CAD build for the part. Positions are in the model's coordinates, mm. A direction names the side the tool comes from. Coordinates: 2 decimals unless noted, no trailing zeros. Write each loop counter-clockwise with the first axis right and the second up, starting at its lowest first coordinate (ties: lowest second). Pieces come first, ordered by that corner, then holes.
```python
from build123d import *

# Parameters (mm, degrees)
F0_W     = 30
F0_H     = 4.3
F1_DEPTH = 4.3
F2_W     = 4
F2_H     = 2.3
F6_DEPTH = 4.301
F3_SIZE  = 0.25
F4_R     = 1.5
F5_DEPTH = 23


with BuildPart() as f1:
    # F0 (on Top) → F1 (new body)
    with BuildSketch(Plane.XY):
        with Locations((-1.762214, 2.15)):
            Rectangle(F0_W, F0_H)
    extrude(amount=F1_DEPTH)

    # F2 (on face) → F6 (cut, through all)
    with BuildSketch(Plane.XY.offset(4.3)):
        with Locations((9.737786, 2.15)):
            Rectangle(F2_W, F2_H)
    extrude(amount=-F6_DEPTH, mode=Mode.SUBTRACT)

    # F3
    f3_edges = [f1.edges().sort_by_distance(p)[0] for p in [
        (13.237786, 2.15, 4.3),
        (-1.762214, 0, 4.3),
        (-1.762214, 4.3, 4.3),
        (13.237786, 0, 2.15),
        (13.237786, 4.3, 2.15),
        (-1.762214, 4.3, 0),
        (13.237786, 2.15, 0),
        (-1.762214, 0, 0),
        (9.737786, 3.3, 0),
        (7.737786, 2.15, 0),
        (9.737786, 1, 0),
        (11.737786, 2.15, 0),
        (7.737786, 2.15, 4.3),
        (11.737786, 2.15, 4.3),
        (9.737786, 3.3, 4.3),
        (9.737786, 1, 4.3),
        (-16.762214, 2.15, 4.3),
        (-16.762214, 0, 2.15),
        (-16.762214, 2.15, 0),
        (-16.762214, 4.3, 2.15),
    ]]
    chamfer(f3_edges, length=F3_SIZE)

    # F4 (on face) → F5 (cut)
    with BuildSketch(Plane(origin=(-16.762214, 0, 0), x_dir=(0, -1, 0), z_dir=(-1, 0, 0))):
        with Locations((-2.15, 2.15)):
            Circle(F4_R)
    extrude(amount=-F5_DEPTH, mode=Mode.SUBTRACT)


solid = f1.part
```
Item 1: Saw through at A-A, the plane x = -13.5. Write the cut outline in (y, z), and give its area (3 significant figures).
Item 2: Which spindle directions (+Z, -Z, +X, -X, +Y, -Y) get a long thin tool onto all of the face, cutting with end or side? Do faces 5 (the flat face through (13.238, 2, 2)), 6 (the flat face through (10, 1, 2)), 7 (the cylindrical face through (-5.4, 1.5, 0.8)). Say none if no direction does.
Item 3: Saw through at C-C, the plane z = 2.15. Write the cut outline in (x, y).
Item 4: Saw through at B-B, the plane y = 2.15. Write the cut outline in (x, z).
Item 5: Saw through at D-D, the plane z = 3.25. Write the cut outline in (x, y).
Item 6: Two-plate mould, pull along Z, no slides. Class faces 1 (the flat face through (6.238, 2, 2)), 2 (the flat face through (10, 3.3, 2)), 3 (the flat face through (-5, 2, 0)), 4 (the flat face through (-5, 2, 4.3)): +Z half, -Z half, draft (parallel to the pull), parting line (faces both ways), or undercut.
Item 7: Wall check: line 1 along X through (y, z) = (1.25, 3.5); line 2 along X through (y, z) = (2.15, 3.1); line 3 along Z through (x, y) = (-9.25, 2.15). Give the ranges that are in metal, low to high.
Working result:
1. outline: (0, 0.25) - (0.25, 0) - (4.05, 0) - (4.3, 0.25) - (4.3, 4.05) - (4.05, 4.3) - (0.25, 4.3) - (0, 4.05) - close; hole circle Ø3 at (2.15, 2.15)
1. area: 11.3 mm2
2. face 5: +Z, -Z, +X, +Y, -Y
2. face 6: +Z, -Z
2. face 7: -X
3. outline: (-16.76, 0.25) - (-16.51, 0) - (12.99, 0) - (13.24, 0.25) - (13.24, 4.05) - (12.99, 4.3) - (-16.51, 4.3) - (-16.76, 4.05) - (-16.76, 3.65) - (6.24, 3.65) - (6.24, 0.65) - (-16.76, 0.65) - close; hole (7.74, 1) - (11.74, 1) - (11.74, 3.3) - (7.74, 3.3) - close
4. outline: (-16.76, 0.25) - (-16.51, 0) - (7.49, 0) - (7.74, 0.25) - (7.74, 4.05) - (7.49, 4.3) - (-16.51, 4.3) - (-16.76, 4.05) - (-16.76, 3.65) - (6.24, 3.65) - (6.24, 0.65) - (-16.76, 0.65) - close; (11.74, 0.25) - (11.99, 0) - (12.99, 0) - (13.24, 0.25) - (13.24, 4.05) - (12.99, 4.3) - (11.99, 4.3) - (11.74, 4.05) - close
5. outline: (-16.76, 0.25) - (-16.51, 0) - (12.99, 0) - (13.24, 0.25) - (13.24, 4.05) - (12.99, 4.3) - (-16.51, 4.3) - (-16.76, 4.05) - (-16.76, 3.17) - (6.24, 3.17) - (6.24, 1.13) - (-16.76, 1.13) - close; hole (7.74, 1) - (11.74, 1) - (11.74, 3.3) - (7.74, 3.3) - close
6. face 1: undercut
6. face 2: draft
6. face 3: -Z half
6. face 4: +Z half
7. line 1: x = -16.76 to 7.74, 11.74 to 13.24
7. line 2: x = 6.24 to 7.74, 11.74 to 13.24
7. line 3: z = 0 to 0.65, 3.65 to 4.3
